For this review, take the finished solid that the model builds, in its own axes (mm). A direction names the side the tool comes from. Give positions to 0.01 mm unless a question says otherwise; leave off trailing zeros. Order: outer loops, then holes, each group sorted by start corner. A loop starts at its lowest first (then second) coordinate and runs counter-clockwise, first axis right, second up. Notation, with made-up numbers: (24, 14.5) - (73, 14.5) arc R21 ccw to (73, 22.5) - close; hole circle Ø11 at (45.5, 87). An arc over 180 degrees is marked (long way). Use a Markdown table: item, result. Add a question column.
1) Clearance check with flat-ended pins moving along their axes: P1, Ø3, axis at y = 76, z = 5, coming from the +X side; P2, Ø1, axis at x = -11.5, y = 55, coming from the -Z side; P3, Ø5, axis at y = 10, z = 15, coming from the -X side; P4, Ø14, axis at x = -1, z = -3.5, coming from the -Y side. State where each tip first meets the part, or that it passes through.
2) We need section C-C on z = -15. Write out the cut boundary in (x, y).
3) We need section D-D on x = -20. Write out the cut boundary in (y, z).
4) Wall thickness on L1, parallel to X at y = 4, z = -3; L2, parallel to X at y = 4, z = 10; L3, parallel to Y at x = -5, z = 17: over which ranges is each line inside the solid? List them lowest first.
5) Machinability: for faces 1 (the face through (-1.126, 6.895, 16.615)), 2 (the face through (0, 11.2, 0)), 3 (the face through (-10, -2, 10)), 4 (the face through (4, 28, -20)), which of the approach directions +Z, -Z, +X, -X, +Y, -Y give a long, thin tool a straight path to every point of the face, cutting with its end or side? Answer none if there is none.
6) We need section B-B on x = -3.5. Write out the cut boundary in (y, z), then the cut area to 3 significant figures.
7) Mouldability with a two-part tool opening along Z and no side actions: class faces 5 (the face through (-20, 3, 0)), 6 (the face through (-25, 6, 8)), 7 (the face through (-18, 3, 8)) as released by +Z, released by -Z, zero draft, split by the parting line, or undercut.
8) We need section A-A on y = 25.5. Write out the cut boundary in (x, z).
```python
from build123d import *

# Parameters (mm, degrees)
SKETCH_1_W           = 20
SKETCH_1_H           = 60
SKETCH_1_R           = 2.6
EXTRUDE_1_DEPTH      = 6
SKETCH_2_W           = 6.1
SKETCH_2_H           = 43.9
SKETCH_2_H_2         = 1.95
SKETCH_2_W_2         = 6.043917029
EXTRUDE_2_DEPTH      = 4
SKETCH_3_R           = 4.9
CUT_EXTRUDE_3_DEPTH  = 3
SKETCH_4_W           = 20
SKETCH_4_H           = 40
EXTRUDE_3_DEPTH      = 69
CUT_EXTRUDE_4_DEPTH  = 75
SKETCH_6_R           = 2.1
CUT_EXTRUDE_5_DEPTH  = 75
CUT_EXTRUDE_6_DEPTH  = 75
SKETCH_13_R          = 3.5
CUT_EXTRUDE_8_DEPTH  = 3
SKETCH_14_R          = 3.5
CUT_EXTRUDE_9_DEPTH  = 3
SKETCH_15_W          = 6.1
SKETCH_15_H          = 1.95
SKETCH_15_W_2        = 6.043917029
CUT_EXTRUDE_10_DEPTH = 4
SKETCH_24_R          = 3.5
CUT_EXTRUDE_14_DEPTH = 15
SKETCH_25_R          = 3.5
CUT_EXTRUDE_15_DEPTH = 15
SKETCH_26_W          = 6.1
SKETCH_26_H          = 43.9
CUT_EXTRUDE_16_DEPTH = 4
SKETCH_27_W          = 20
SKETCH_27_H          = 10
CUT_EXTRUDE_17_DEPTH = 10
EXTRUDE_4_DEPTH      = 4
SKETCH_29_R          = 3.5
CUT_EXTRUDE_18_DEPTH = 18
EXTRUDE_5_DEPTH      = 8
SKETCH_31_W          = 20
SKETCH_31_H          = 20
EXTRUDE_6_DEPTH      = 3
CUT_EXTRUDE_19_DEPTH = 6
SKETCH_33_W          = 20
SKETCH_33_H          = 20
SKETCH_33_R          = 5
EXTRUDE_7_DEPTH      = 3


with BuildPart() as part:
    # 草图1 → 凸台-拉伸1 (new body)
    with BuildSketch(Plane(origin=(0, 0, 0), x_dir=(1, 0, 0), z_dir=(0, 1, 0))):
        Rectangle(SKETCH_1_W, SKETCH_1_H)
        with Locations(Location((0, 25, 0), (0, 0, 270))):
            Circle(SKETCH_1_R, mode=Mode.SUBTRACT)
        with Locations(Location((0, -25, 0), (0, 0, 270))):
            Circle(SKETCH_1_R, mode=Mode.SUBTRACT)
    extrude(amount=EXTRUDE_1_DEPTH)

    # 草图2 → 凸台-拉伸2 (add)
    with BuildSketch(Plane.XZ):
        Rectangle(SKETCH_2_W, SKETCH_2_H)
        with Locations((0, 29.025)):
            Rectangle(SKETCH_2_W, SKETCH_2_H_2)
        with Locations((0.028041485, -29.025)):
            Rectangle(SKETCH_2_W_2, SKETCH_2_H_2)
    extrude(amount=EXTRUDE_2_DEPTH)

    # 草图3 → 切除-拉伸3 (cut)
    with BuildSketch(Plane(origin=(0, 6, 0), x_dir=(1, 0, 0), z_dir=(0, 1, 0))):
        with Locations(Location((0, -25, 0), (0, 0, 270))):
            Circle(SKETCH_3_R)
        with Locations(Location((0, 25, 0), (0, 0, 270))):
            Circle(SKETCH_3_R)
    extrude(amount=-CUT_EXTRUDE_3_DEPTH, mode=Mode.SUBTRACT)

    # 草图4 → 凸台-拉伸3 (add)
    with BuildSketch(Plane(origin=(0, 6, 0), x_dir=(1, 0, 0), z_dir=(0, 1, 0))):
        Rectangle(SKETCH_4_W, SKETCH_4_H)
    extrude(amount=EXTRUDE_3_DEPTH)

    # 草图5 → 切除-拉伸4 (cut)
    with BuildSketch(Plane.ZY.offset(10)):
        Polygon((-8.8, 11.2), (0, 11.2), (8.8, 11.2), (8.8, 28.8), (0, 28.8), (-8.8, 28.8), align=None)
    extrude(amount=-CUT_EXTRUDE_4_DEPTH, mode=Mode.SUBTRACT)

    # 草图6 → 切除-拉伸5 (cut)
    with BuildSketch(Plane.ZY.offset(10)):
        with Locations((0, 70)):
            Circle(SKETCH_6_R)
        with Locations((-15, 10)):
            Circle(SKETCH_6_R)
        with Locations((15, 10)):
            Circle(SKETCH_6_R)
    extrude(amount=-CUT_EXTRUDE_5_DEPTH, mode=Mode.SUBTRACT)

    # 草图7 → 切除-拉伸6 (cut)
    with BuildSketch(Plane.ZY.offset(10)):
        with BuildLine():
            Line((-20, 75), (-20, 55))
            ThreePointArc((-20, 55), (-14.142135624, 69.142135624), (0, 75))
            Line((0, 75), (-20, 75))
        make_face()
        with BuildLine():
            Line((20, 75), (0, 75))
            ThreePointArc((0, 75), (14.142135624, 69.142135624), (20, 55))
            Line((20, 55), (20, 75))
        make_face()
    extrude(amount=-CUT_EXTRUDE_6_DEPTH, mode=Mode.SUBTRACT)

    # 草图13 → 切除-拉伸8 (cut)
    with BuildSketch(Plane.ZY.offset(10)):
        with Locations((-15, 10)):
            Circle(SKETCH_13_R)
        with Locations((15, 10)):
            Circle(SKETCH_13_R)
    extrude(amount=-CUT_EXTRUDE_8_DEPTH, mode=Mode.SUBTRACT)

    # 草图14 → 切除-拉伸9 (cut)
    with BuildSketch(Plane.ZY.offset(-5)):
        with Locations(Location((0, 70, 0), (0, 0, 270))):
            Circle(SKETCH_14_R)
    extrude(amount=-CUT_EXTRUDE_9_DEPTH, mode=Mode.SUBTRACT)

    # 草图15 → 切除-拉伸10 (cut)
    with BuildSketch(Plane(origin=(0, -4, 0), x_dir=(-1, 0, 0), z_dir=(0, -1, 0))):
        with Locations((0, -29.025)):
            Rectangle(SKETCH_15_W, SKETCH_15_H)
        with Locations((-0.028041485, 29.025)):
            Rectangle(SKETCH_15_W_2, SKETCH_15_H)
    extrude(amount=-CUT_EXTRUDE_10_DEPTH, mode=Mode.SUBTRACT)

    # 草图24 → 切除-拉伸14 (cut)
    with BuildSketch(Plane.ZY.offset(10)):
        with Locations((-15, 10)):
            Circle(SKETCH_24_R)
        with Locations((15, 10)):
            Circle(SKETCH_24_R)
    extrude(amount=-CUT_EXTRUDE_14_DEPTH, mode=Mode.SUBTRACT)

    # 草图25 → 切除-拉伸15 (cut)
    with BuildSketch(Plane.ZY.offset(10)):
        with Locations(Location((0, 70, 0), (0, 0, 270))):
            Circle(SKETCH_25_R)
    extrude(amount=-CUT_EXTRUDE_15_DEPTH, mode=Mode.SUBTRACT)

    # 草图26 → 切除-拉伸16 (cut)
    with BuildSketch(Plane(origin=(0, -4, 0), x_dir=(-1, 0, 0), z_dir=(0, -1, 0))):
        Rectangle(SKETCH_26_W, SKETCH_26_H)
    extrude(amount=-CUT_EXTRUDE_16_DEPTH, mode=Mode.SUBTRACT)

    # 草图27 → 切除-拉伸17 (cut)
    with BuildSketch(Plane(origin=(0, 6, 0), x_dir=(1, 0, 0), z_dir=(0, 1, 0))):
        with Locations((0, 25)):
            Rectangle(SKETCH_27_W, SKETCH_27_H)
        with Locations((0, -25)):
            Rectangle(SKETCH_27_W, SKETCH_27_H)
    extrude(amount=-CUT_EXTRUDE_17_DEPTH, mode=Mode.SUBTRACT)

    # 草图28 → 凸台-拉伸4 (add)
    with BuildSketch(Plane.XZ):
        Polygon((10, 6.95), (10, 10), (10, 13.05), (-10, 13.05), (-10, 10), (-10, 6.95), align=None)
    extrude(amount=EXTRUDE_4_DEPTH)

    # 草图29 → 切除-拉伸18 (cut)
    with BuildSketch(Plane.ZY.offset(10)):
        with Locations(Location((0, 70, 0), (0, 0, 270))):
            Circle(SKETCH_29_R)
        with Locations((15, 10)):
            Circle(SKETCH_29_R)
        with Locations((-15, 10)):
            Circle(SKETCH_29_R)
    extrude(amount=-CUT_EXTRUDE_18_DEPTH, mode=Mode.SUBTRACT)

    # 草图30 → 凸台-拉伸5 (add)
    with BuildSketch(Plane.ZY.offset(10)):
        with BuildLine():
            Line((20, 55), (20, 89))
            Line((20, 89), (0, 89))
            Line((0, 89), (-21, 65))
            Line((-21, 65), (-21, 0))
            Line((-21, 0), (-20, 0))
            Line((-20, 0), (-20, 55))
            ThreePointArc((-20, 55), (0, 75), (20, 55))
        make_face()
    extrude(amount=-EXTRUDE_5_DEPTH)

    # 草图31 → 凸台-拉伸6 (add)
    with BuildSketch(Plane.XZ):
        with Locations((-20, 10)):
            Rectangle(SKETCH_31_W, SKETCH_31_H)
    extrude(amount=-EXTRUDE_6_DEPTH)

    # 草图32 → 切除-拉伸19 (cut)
    with BuildSketch(Plane(origin=(0, 0, 0), x_dir=(-1, 0, 0), z_dir=(0, -1, 0))):
        with BuildLine():
            ThreePointArc((18.161522369, -8.161522369), (18.161522369, -11.838477631), (21.838477631, -11.838477631))
            Line((21.838477631, -11.838477631), (18.161522369, -8.161522369))
        make_face()
        with BuildLine():
            Line((18.161522369, -8.161522369), (21.838477631, -11.838477631))
            ThreePointArc((21.838477631, -11.838477631), (22.402086785, -10.994976924), (22.6, -10))
            ThreePointArc((22.6, -10), (20.994976924, -7.597913215), (18.161522369, -8.161522369))
        make_face()
    extrude(amount=-CUT_EXTRUDE_19_DEPTH, mode=Mode.SUBTRACT)

    # 草图33 → 凸台-拉伸7 (add)
    with BuildSketch(Plane(origin=(0, 3, 0), x_dir=(1, 0, 0), z_dir=(0, 1, 0))):
        with Locations((-20, -10)):
            Rectangle(SKETCH_33_W, SKETCH_33_H)
        with Locations(Location((-20, -10, 0), (0, 0, 270))):
            Circle(SKETCH_33_R, mode=Mode.SUBTRACT)
    extrude(amount=EXTRUDE_7_DEPTH)


solid = part.part
```
Checked values:
| question | item | result |
|---|---|---|
| 1 | P1 | x = -2 |
| 1 | P2 | through |
| 1 | P3 | x = 8 |
| 1 | P4 | y = 0 |
| 2 | outline | (-10, 0) - (10, 0) - (10, 7.9) - (8, 7.9) - (8, 6.5) - (-10, 6.5) - close; (-10, 13.5) - (8, 13.5) - (8, 12.1) - (10, 12.1) - (10, 68.23) - (-2, 68.23) - (-2, 71.86) - (-10, 71.86) - close |
| 3 | outline | (0, 0) - (6, 0) - (6, 5) - (3, 5) - (3, 7.4) - (0, 7.4) - close; (0, 12.6) - (3, 12.6) - (3, 15) - (6, 15) - (6, 20) - (0, 20) - close |
| 4 | L1 | -10 to 10 |
| 4 | L2 | -30 to -25, -15 to 10 |
| 4 | L3 | 0 to 7.13, 12.87 to 89 |
| 5 | face 1 | -X |
| 5 | face 2 | +X, -X |
| 5 | face 3 | +Z, -Z, -X, -Y |
| 5 | face 4 | -Z, +X, +Y, -Y |
| 6 | outline | (-4, 6.95) - (0, 6.95) - (0, -21) - (65, -21) - (89, 0) - (89, 20) - (0, 20) - (0, 13.05) - (-4, 13.05) - close; hole circle Ø7 at (10, -15); hole circle Ø7 at (10, 15); hole (11.2, -8.8) - (28.8, -8.8) - (28.8, 8.8) - (11.2, 8.8) - close; hole circle Ø7 at (70, 0) |
| 6 | area | 3,000 mm² |
| 7 | face 5 | released by -Z |
| 7 | face 6 | zero draft |
| 7 | face 7 | undercut |
| 8 | outline | (-10, -21) - (-2, -21) - (-2, -20) - (10, -20) - (10, -8.8) - (-10, -8.8) - close; (-10, 8.8) - (10, 8.8) - (10, 20) - (-10, 20) - close |
